Design review of the part built by this model. Coordinates are the model's own, in mm. A direction names the side the tool comes from. Round coordinates to 2 decimals unless told otherwise and drop trailing zeros. Loops run counter-clockwise (first coordinate to the right, second up) from the corner with the lowest first, then second, coordinate; pieces in that order, holes last. Notation, with made-up numbers: (10, 72.5) - (24, 72.5) arc R23 cw to (24, 90.5) - close; hole circle Ø10 at (36.5, -24). An arc over 180 degrees is marked (long way). Answer as CSV lines item,"result". Start each with the question number.
(1) For faces 4 (the flat face through (20, 0, -10)), 5 (the flat face through (40.5, -3, -10.3)), 6 (the flat face through (-1, -3, -10)), 7 (the cylindrical face through (12, 2, -2)), list the 3-axis set-ups (+Z, -Z, +X, -X, +Y, -Y) from which the entire face can be reached by the end or side of a thin tool; tool diameter is ignored.
(2) Mouldability with a two-part tool opening along X and no side actions: class faces 1 (the flat face through (40, -4, -23)), 2 (the flat face through (19, -1, -26)), 3 (the flat face through (0, -2, -10)) as released by +X, released by -X, zero draft, split by the parting line, or undercut.
(3) Wall thickness on L1, parallel to X at y = 1.55, z = -16.5; L2, parallel to X at y = 1, z = 2.5; L3, parallel to Z at x = 7, y = -3.5: over which ranges is each line inside the solid? List them lowest first.
(4) Consider section A-A (y = -3.75). Give the boundary of the cut face in (x, z).
(5) Consider section B-B (x = 12). Give the boundary of the cut face in (y, z).
(6) For P1, Ø1, axis at y = -4.5, z = -23.5, coming from the -X side; P2, Ø4, axis at x = 15.5, z = -14.5, coming from the -Y side; P3, Ø1.6, axis at y = -4.5, z = 3.5, coming from the +X side, all flat-tipped, find the tip position at first contact; note any pin that passes through.
(7) Consider section C-C (z = 2.5). Give the boundary of the cut face in (x, y), and give its area (3 significant figures).
(8) Consider section D-D (x = 28). Give the boundary of the cut face in (y, z).
from build123d import *

# Parameters (mm, degrees)
SKETCH_1_W          = 40
SKETCH_1_H          = 20
EXTRUDE_1_DEPTH     = 3
SKETCH_2_R          = 1.5
CUT_EXTRUDE_1_DEPTH = 3
SKETCH_3_W          = 40
SKETCH_3_H          = 8
EXTRUDE_2_DEPTH     = 5
SKETCH_4_W          = 40
SKETCH_4_H          = 8
EXTRUDE_3_DEPTH     = 6
SKETCH_6_R          = 1.3
CUT_EXTRUDE_2_DEPTH = 8
SKETCH_11_W         = 1.5
SKETCH_11_H         = 6
EXTRUDE_5_DEPTH     = 31
SKETCH_12_W         = 31
SKETCH_12_H         = 6
EXTRUDE_6_DEPTH     = 1


with BuildPart() as part:
    # 草圖1 → 填料-伸長1 (new body)
    with BuildSketch(Plane(origin=(0, 0, 0), x_dir=(1, 0, 0), z_dir=(0, 1, 0))):
        with Locations((20, 10)):
            Rectangle(SKETCH_1_W, SKETCH_1_H)
    extrude(amount=EXTRUDE_1_DEPTH)

    # 草圖2 → 除料-伸長1 (cut)
    with BuildSketch(Plane(origin=(0, 3, 0), x_dir=(1, 0, 0), z_dir=(0, 1, 0))):
        with Locations(Location((28, 16.5, 0), (0, 0, 270))):
            Circle(SKETCH_2_R)
        with Locations(Location((12, 16.5, 0), (0, 0, 270))):
            Circle(SKETCH_2_R)
        with Locations(Location((12, 3.5, 0), (0, 0, 270))):
            Circle(SKETCH_2_R)
        with Locations(Location((28, 3.5, 0), (0, 0, 270))):
            Circle(SKETCH_2_R)
    extrude(amount=-CUT_EXTRUDE_1_DEPTH, mode=Mode.SUBTRACT)

    # 草圖3 → 填料-伸長2 (add)
    with BuildSketch(Plane.XY):
        with Locations((20, -1)):
            Rectangle(SKETCH_3_W, SKETCH_3_H)
    extrude(amount=EXTRUDE_2_DEPTH)

    # 草圖4 → 填料-伸長3 (add)
    with BuildSketch(Plane(origin=(0, 0, -20), x_dir=(-1, 0, 0), z_dir=(0, 0, -1))):
        with Locations((-20, -1)):
            Rectangle(SKETCH_4_W, SKETCH_4_H)
    extrude(amount=EXTRUDE_3_DEPTH)

    # 草圖6 → 除料-伸長2 (cut)
    with BuildSketch(Plane(origin=(0, 3, 0), x_dir=(1, 0, 0), z_dir=(0, 1, 0))):
        with Locations(Location((8.5, 23.5, 0), (0, 0, 270))):
            Circle(SKETCH_6_R)
        with Locations(Location((18.5, 23.5, 0), (0, 0, 270))):
            Circle(SKETCH_6_R)
        with Locations(Location((28.5, 23.5, 0), (0, 0, 270))):
            Circle(SKETCH_6_R)
        with Locations(Location((8.5, -2.5, 0), (0, 0, 270))):
            Circle(SKETCH_6_R)
        with Locations(Location((18.5, -2.5, 0), (0, 0, 270))):
            Circle(SKETCH_6_R)
        with Locations(Location((28.5, -2.5, 0), (0, 0, 270))):
            Circle(SKETCH_6_R)
    extrude(amount=-CUT_EXTRUDE_2_DEPTH, mode=Mode.SUBTRACT)

    # 草圖11 → 填料-伸長5 (add)
    with BuildSketch(Plane.XY.offset(5)):
        with Locations((-0.75, 0)):
            Rectangle(SKETCH_11_W, SKETCH_11_H)
    extrude(amount=-EXTRUDE_5_DEPTH)

    # 草圖12 → 填料-伸長6 (add)
    with BuildSketch(Plane(origin=(40, 0, 0), x_dir=(0, 0, -1), z_dir=(1, 0, 0))):
        with Locations((10.5, 0)):
            Rectangle(SKETCH_12_W, SKETCH_12_H)
    extrude(amount=EXTRUDE_6_DEPTH)


solid = part.part
Determined:
1,face 4,"-Y"
1,face 5,"+Z, -Z, +X, -Y"
1,face 6,"+Z, -Z, -X, -Y"
1,face 7,"+Y, -Y"
2,face 1,"released by +X"
2,face 2,"zero draft"
2,face 3,"undercut"
3,L1,"x = -1.5 to 10.5, 13.5 to 26.5, 29.5 to 41"
3,L2,"x = -1.5 to 7.2, 9.8 to 17.2, 19.8 to 27.2, 29.8 to 41"
3,L3,"z = -26 to -20, 0 to 5"
4,outline,"(0, -26) - (40, -26) - (40, -20) - (0, -20) - close; (0, 0) - (40, 0) - (40, 5) - (0, 5) - close; hole circle Ø2.6 at (8.5, -23.5); hole circle Ø2.6 at (8.5, 2.5); hole circle Ø2.6 at (18.5, -23.5); hole circle Ø2.6 at (18.5, 2.5); hole circle Ø2.6 at (28.5, -23.5); hole circle Ø2.6 at (28.5, 2.5)"
5,outline,"(-5, -26) - (3, -26) - (3, -18) - (0, -18) - (0, -20) - (-5, -20) - close; (-5, 0) - (0, 0) - (0, -2) - (3, -2) - (3, 5) - (-5, 5) - close; (0, -15) - (3, -15) - (3, -5) - (0, -5) - close"
6,P1,"stops at x = 0"
6,P2,"stops at y = 0"
6,P3,"stops at x = 40"
7,outline,"(-1.5, -3) - (0, -3) - (0, -5) - (7.2, -5) - (7.2, 3) - (-1.5, 3) - close; (9.8, -5) - (17.2, -5) - (17.2, 3) - (9.8, 3) - close; (19.8, -5) - (27.2, -5) - (27.2, 3) - (19.8, 3) - close; (29.8, -5) - (40, -5) - (40, -3) - (41, -3) - (41, 3) - (29.8, 3) - close"
7,area,"273 mm^2"
8,outline,"(-5, -26) - (3, -26) - (3, -24.7) - (-5, -24.7) - close; (-5, -22.3) - (3, -22.3) - (3, -18) - (0, -18) - (0, -20) - (-5, -20) - close; (-5, 0) - (0, 0) - (0, -2) - (3, -2) - (3, 1.3) - (-5, 1.3) - close; (-5, 3.7) - (3, 3.7) - (3, 5) - (-5, 5) - close; (0, -15) - (3, -15) - (3, -5) - (0, -5) - close"
